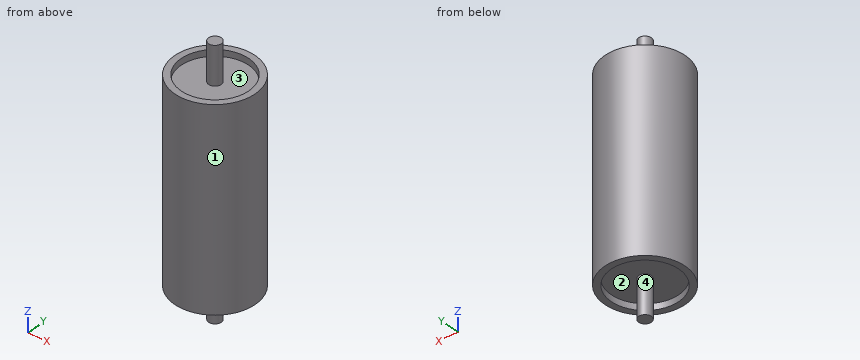
Autodesk Inventor part; units mm, degrees
ref_plane "YZ Plane" through (0, 0, 0) normal (1, 0, 0) x (0, 1, 0)
ref_plane "XZ Plane" through (0, 0, 0) normal (0, 1, 0) x (-1, 0, 0)
ref_plane "XY Plane" through (0, 0, 0) normal (0, 0, 1) x (1, 0, 0)
sketch "Sketch1" plane through (0, 0, 0) normal (0, 0, 1) x (1, 0, 0)
  circle A0 centre (0, 0) radius 31.75
  dimension "d0" = 31.75
extrude "Extrusion1" add sketch "Sketch1" along normal mid plane 155
sketch "Sketch2" plane through (0, 0, -77.5) normal (0, 0, -1) x (-1, 0, 0)
  circle A0 centre (0, 0) radius 26.75
  dimension "d3" = 26.75
extrude "Extrusion2" cut sketch "Sketch2" against normal blind 5
sketch "Sketch3" plane through (0, 0, 77.5) normal (0, 0, 1) x (1, 0, 0)
  circle A0 centre (0, 0) radius 26.75
  dimension "d6" = 26.75
extrude "Extrusion3" cut sketch "Sketch3" against normal blind 5
sketch "Sketch4" plane through (0, 0, -72.5) normal (0, 0, -1) x (-1, 0, 0)
  circle A0 centre (0, 0) radius 5
  dimension "d9" = 5
extrude "Extrusion4" add sketch "Sketch4" along normal blind 30
sketch "Sketch5" plane through (0, 0, 72.5) normal (0, 0, 1) x (1, 0, 0)
  circle A0 centre (0, 0) radius 5
  dimension "d12" = 5
extrude "Extrusion5" add sketch "Sketch5" along normal blind 30
properties part number "Rodo"
CAD build for the part. Positions are in the model's coordinates, mm. Face numbers are marked on the shaded views. A direction names the side the tool comes from. Give positions to 0.01 mm unless a question says otherwise; leave off trailing zeros. Order: outer loops, then holes, each group sorted by start corner. A loop starts at its lowest first (then second) coordinate and runs counter-clockwise, first axis right, second up. Notation, with made-up numbers: (17, 45.5) - (32, 45.5) arc R13 cw to (32, 49.5) - close; hole circle Ø11 at (30.25, 20.5). An arc over 180 degrees is marked (long way). Write each question's results on one line, items separated by ' | '.
1. Saw through at C-C on z = -67. List the corners of the cut face in (x, y), and give its area (3 significant figures).
Calculated:
outline: circle Ø63.5 at (0, 0) | area: 3,170 mm2
2. 3-axis set-ups, long thin cutter, end or side, ignore diameter. For the marked faces 3 and 4: which of +Z, -Z, +X, -X, +Y, -Y reach the whole face in a straight line?
Calculated:
face 3: +Z | face 4: -Z
3. Probe L1, parallel to Y at x = 0, z = -74.75; L2, parallel to Z at x = -16.5, y = -18.5; L3, parallel to Y at x = -13, z = 49. List the from-to ranges inside material, lowest first. Write a range as from..to.
Calculated:
L1: y = -31.75..-26.75, -5..5, 26.75..31.75 | L2: z = -72.5..72.5 | L3: y = -28.97..28.97
4. Pull direction Y, two halves, no side cores. Call the marked faces 1 and 2: released by +Y, released by -Y, zero draft, split by the parting line, or undercut.
Calculated:
face 1: split by the parting line | face 2: undercut
5. Saw through at D-D on y = -15.5. List the corners of the cut face in (x, z).
Calculated:
outline: (-27.71, -77.5) - (-21.8, -77.5) - (-21.8, -72.5) - (21.8, -72.5) - (21.8, -77.5) - (27.71, -77.5) - (27.71, 77.5) - (21.8, 77.5) - (21.8, 72.5) - (-21.8, 72.5) - (-21.8, 77.5) - (-27.71, 77.5) - close
6. Saw through at A-A on y = 0. List the corners of the cut face in (x, z), and give its area (3 significant figures).
Calculated:
outline: (-31.75, -77.5) - (-26.75, -77.5) - (-26.75, -72.5) - (-5, -72.5) - (-5, -102.5) - (5, -102.5) - (5, -72.5) - (26.75, -72.5) - (26.75, -77.5) - (31.75, -77.5) - (31.75, 77.5) - (26.75, 77.5) - (26.75, 72.5) - (5, 72.5) - (5, 102.5) - (-5, 102.5) - (-5, 72.5) - (-26.75, 72.5) - (-26.75, 77.5) - (-31.75, 77.5) - close | area: 9,910 mm2
7. Pin check, flat tips, straight feed: pin 1 (1.5 mm diameter, centred on x = 20, y = 11, fed in from +Z); pin 2 (4 mm diameter, centred on x = 23, y = 16.5, fed in from -Z); pin 3 (1.5 mm diameter, centred on x = -11.5, z = -33, fed in from -Y). Stop position of each tip, or through.
Calculated:
pin 1: stops at z = 72.5 | pin 2: stops at z = -77.5 | pin 3: stops at y = -29.87
